For this review, take the finished solid that the model builds, in its own axes (mm). Face numbers are marked on the shaded views. A direction names the side the tool comes from. Coordinates: 2 decimals unless noted, no trailing zeros. Order: outer loops, then holes, each group sorted by start corner. A loop starts at its lowest first (then second) coordinate and runs counter-clockwise, first axis right, second up.
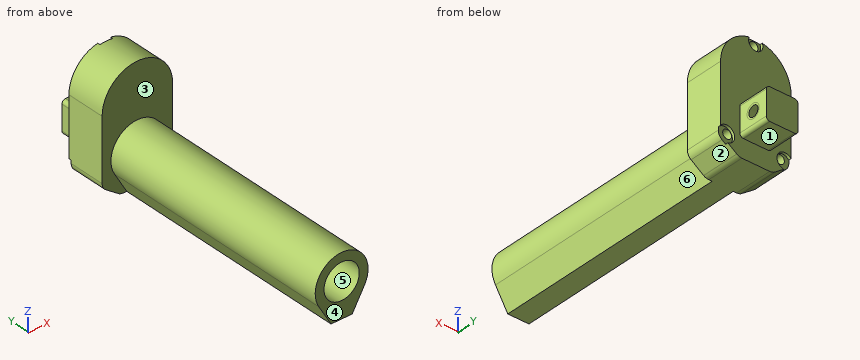
from build123d import *

# Parameters (mm, degrees)
SALIENTE_EXTRUIR1_DEPTH = 22
CROQUIS3_R              = 4.5
CROQUIS3_R_2            = 2.5
CORTAR_EXTRUIR2_DEPTH   = 1.5
CROQUIS4_R              = 2.5
CORTAR_EXTRUIR3_DEPTH   = 18
CROQUIS5_R              = 4.05861195
CORTAR_EXTRUIR4_DEPTH   = 1.5
CROQUIS6_R              = 2.5
CORTAR_EXTRUIR5_DEPTH   = 15
SALIENTE_EXTRUIR2_DEPTH = 19
CROQUIS8_R              = 3
CORTAR_EXTRUIR7_DEPTH   = 19
CROQUIS9_R              = 4
CORTAR_EXTRUIR10_DEPTH  = 0.5
CORTAR_EXTRUIR10_DRAFT  = -80
CROQUIS10_R             = 4
CORTAR_EXTRUIR11_DEPTH  = 0.5
CORTAR_EXTRUIR11_DRAFT  = -80
SALIENTE_EXTRUIR3_DEPTH = 135.5
CROQUIS12_R             = 10
CORTAR_EXTRUIR12_DEPTH  = 100


with BuildPart() as part:
    # Croquis2 → Saliente-Extruir1 (new body)
    with BuildSketch(Plane(origin=(0, 0, 0), x_dir=(1, 0, 0), z_dir=(0, 1, 0))):
        with BuildLine():
            Line((-17.906190969, 38.99557788), (-10.803865702, 44.068667356))
            ThreePointArc((-10.803865702, 44.068667356), (-9.423561888, 44.761477543), (-7.897674733, 45))
            Line((-7.897674733, 45), (7.897674733, 45))
            ThreePointArc((7.897674733, 45), (9.423561888, 44.761477543), (10.803865702, 44.068667356))
            Line((10.803865702, 44.068667356), (17.906190969, 38.99557788))
            ThreePointArc((17.906190969, 38.99557788), (19.445838214, 37.214818428), (20, 34.926910524))
            Line((20, 34.926910524), (20, 0))
            ThreePointArc((20, 0), (0, -20), (-20, 0))
            Line((-20, 0), (-20, 34.926910524))
            ThreePointArc((-20, 34.926910524), (-19.445838214, 37.214818428), (-17.906190969, 38.99557788))
        make_face()
    extrude(amount=SALIENTE_EXTRUIR1_DEPTH)

    # Croquis3 → Cortar-Extruir2 (cut)
    # profile 1 of 2: a face of its own
    with BuildSketch(Plane(origin=(0, 22, 0), x_dir=(1, 0, 0), z_dir=(0, 1, 0))):
        with Locations((-16.5, 36)):
            Circle(CROQUIS3_R)
        with Locations(Location((-15, 34.926910524, 0), (0, 0, 270))):
            Circle(CROQUIS3_R_2, mode=Mode.SUBTRACT)
    # profile 2 of 2: a face of its own
    with BuildSketch(Plane(origin=(0, 22, 0), x_dir=(1, 0, 0), z_dir=(0, 1, 0))):
        with Locations((16.5, 36)):
            Circle(CROQUIS3_R)
        with Locations(Location((15, 34.926910524, 0), (0, 0, 270))):
            Circle(CROQUIS3_R_2, mode=Mode.SUBTRACT)
    extrude(amount=-CORTAR_EXTRUIR2_DEPTH, mode=Mode.SUBTRACT)

    # Croquis4 → Cortar-Extruir3 (cut)
    with BuildSketch(Plane(origin=(0, 22, 0), x_dir=(1, 0, 0), z_dir=(0, 1, 0))):
        with Locations(Location((-15, 34.926910524, 0), (0, 0, 270))):
            Circle(CROQUIS4_R)
        with Locations(Location((15, 34.926910524, 0), (0, 0, 270))):
            Circle(CROQUIS4_R)
    extrude(amount=-CORTAR_EXTRUIR3_DEPTH, mode=Mode.SUBTRACT)

    # Croquis5 → Cortar-Extruir4 (cut)
    with BuildSketch(Plane(origin=(0, 22, 0), x_dir=(1, 0, 0), z_dir=(0, 1, 0))):
        with Locations((0.022007055, -18)):
            Circle(CROQUIS5_R)
    extrude(amount=-CORTAR_EXTRUIR4_DEPTH, mode=Mode.SUBTRACT)

    # Croquis6 → Cortar-Extruir5 (cut)
    with BuildSketch(Plane(origin=(0, 20.5, 0), x_dir=(1, 0, 0), z_dir=(0, 1, 0))):
        with Locations(Location((0.024452265, -16.999985052, 0), (0, 0, 270))):
            Circle(CROQUIS6_R)
    extrude(amount=-CORTAR_EXTRUIR5_DEPTH, mode=Mode.SUBTRACT)

    # Croquis7 → Saliente-Extruir2 (add)
    with BuildSketch(Plane(origin=(0, 20.5, 0), x_dir=(1, 0, 0), z_dir=(0, 1, 0))):
        with BuildLine():
            Line((7.003665578, 16.460210879), (-7.003665578, 16.460210879))
            ThreePointArc((-7.003665578, 16.460210879), (-8.41787914, 17.045997317), (-9.003665578, 18.460210879))
            Line((-9.003665578, 18.460210879), (-9.003665578, 32.465325191))
            ThreePointArc((-9.003665578, 32.465325191), (-8.41787914, 33.879538753), (-7.003665578, 34.465325191))
            Line((-7.003665578, 34.465325191), (7.003665578, 34.465325191))
            ThreePointArc((7.003665578, 34.465325191), (8.41787914, 33.879538753), (9.003665578, 32.465325191))
            Line((9.003665578, 32.465325191), (9.003665578, 18.460210879))
            ThreePointArc((9.003665578, 18.460210879), (8.41787914, 17.045997317), (7.003665578, 16.460210879))
        make_face()
    extrude(amount=SALIENTE_EXTRUIR2_DEPTH)

    # Croquis8 → Cortar-Extruir7 (cut)
    with BuildSketch(Plane.ZY.offset(9.003665578)):
        with Locations((-25.462768035, 30.75)):
            Circle(CROQUIS8_R)
    extrude(amount=-CORTAR_EXTRUIR7_DEPTH, mode=Mode.SUBTRACT)


with BuildPart() as cortar_extruir10_tool:
    # Croquis9 → Cortar-Extruir10 (with draft: the straight prism first)
    with BuildSketch(Plane.ZY.offset(9.003665578)):
        with Locations((-25.462768035, 30.75)):
            Circle(CROQUIS9_R)
    extrude(amount=-CORTAR_EXTRUIR10_DEPTH)
    # Cortar-Extruir10: the draft: its side faces are tilted about the plane it starts from
    cortar_extruir10_sides = [cortar_extruir10_tool.faces().sort_by_distance(p)[0] for p in [
        (-8.753665578, 30.75, -29.462768035),
    ]]
    draft(cortar_extruir10_sides, Plane.ZY.offset(9.003665578), CORTAR_EXTRUIR10_DRAFT)


with BuildPart() as part_1:
    add(part.part)

    # Cortar-Extruir10: cut by cortar_extruir10_tool
    add(cortar_extruir10_tool.part, mode=Mode.SUBTRACT)


with BuildPart() as cortar_extruir11_tool:
    # Croquis10 → Cortar-Extruir11 (with draft: the straight prism first)
    with BuildSketch(Plane(origin=(9.003665578, 0, 0), x_dir=(0, 0, -1), z_dir=(1, 0, 0))):
        with Locations((25.462768035, 30.75)):
            Circle(CROQUIS10_R)
    extrude(amount=-CORTAR_EXTRUIR11_DEPTH)
    # Cortar-Extruir11: the draft: its side faces are tilted about the plane it starts from
    cortar_extruir11_sides = [cortar_extruir11_tool.faces().sort_by_distance(p)[0] for p in [
        (8.753665578, 30.75, -21.462768035),
    ]]
    draft(cortar_extruir11_sides, Plane(origin=(9.003665578, 0, 0), x_dir=(0, 0, -1), z_dir=(1, 0, 0)), CORTAR_EXTRUIR11_DRAFT)


with BuildPart() as part_2:
    add(part_1.part)

    # Cortar-Extruir11: cut by cortar_extruir11_tool
    add(cortar_extruir11_tool.part, mode=Mode.SUBTRACT)

    # Croquis11 → Saliente-Extruir3 (add)
    with BuildSketch(Plane.XZ):
        with BuildLine():
            Line((-6, -45), (-12.97133054, -32.995668142))
            ThreePointArc((-12.97133054, -32.995668142), (0, -10.462768035), (12.97133054, -32.995668142))
            Line((12.97133054, -32.995668142), (6, -45))
            Line((6, -45), (-6, -45))
        make_face()
    extrude(amount=SALIENTE_EXTRUIR3_DEPTH)

    # Croquis12 → Cortar-Extruir12 (cut)
    with BuildSketch(Plane.XZ.offset(135.5)):
        with Locations(Location((0, -25.462768035, 0), (0, 0, 270))):
            Circle(CROQUIS12_R)
    extrude(amount=-CORTAR_EXTRUIR12_DEPTH, mode=Mode.SUBTRACT)


solid = part_2.part
1. Take a section at C-C, the plane z = -13.5. Give the boundary of the cut face in (x, y), plus the area to 3 significant figures.
Answer below:
outline: (-20, 0) - (-9.05, 0) - (-9.05, -135.5) - (9.05, -135.5) - (9.05, 0) - (20, 0) - (20, 22) - (-20, 22) - close
area: 3,330 mm2
2. Take a section at A-A, the plane y = -123. Give the boundary of the cut face in (x, z), plus the area to 3 significant figures.
Answer below:
outline: (-12.97, -33) - (-6, -45) - (6, -45) - (12.97, -33) arc R15 ccw (long way) to start; hole circle Ø20 at (0, -25.46)
area: 483 mm2
3. Take a section at B-B, the plane z = 12. Give the boundary of the cut face in (x, y), plus the area to 3 significant figures.
Answer below:
outline: (-16, 0) - (16, 0) - (16, 22) - (-16, 22) - close
area: 704 mm2
4. The part is to be moulded in two halves that separate along Z. For the marked faces 4, 5 and 6, say which applies: +Z half, -Z half, draft (parallel to the pull), parting line (faces both ways), or undercut.
Answer below:
face 4: draft
face 5: undercut
face 6: -Z half
5. Machinability: for the marked faces 1, 2 and 3, which of the approach directions +Z, -Z, +X, -X, +Y, -Y give a long, thin tool a straight path to every point of the face, cutting with its end or side? Answer none if there is none.
Answer below:
face 1: -Z, +X, -X, +Y
face 2: -Z, +X, +Y, -Y
face 3: -Y
6. Clearance check with flat-ended pins moving along their axes: pin 1 Ø1.5 at (x, z) = (15, -36) entering from +Y; pin 2 Ø15.5 at (y, z) = (30.5, -23.5) entering from +X; pin 3 Ø1.5 at (x, z) = (-1, 17) entering from +Y. State where each tip first meets the part, or that it passes through.
Answer below:
pin 1: stops at y = 4
pin 2: stops at x = 9
pin 3: stops at y = 5.5
7. To check wall thickness, follow L1, parallel to Z at x = -0.5, y = -99; L2, parallel to Y at x = -4, z = 4; L3, parallel to Y at x = 12, z = -29. State the ranges of each line that lie inside material, in increasing order.
Answer below:
L1: z = -45 to -35.45, -15.48 to -10.47
L2: y = 0 to 22
L3: y = -135.5 to 22
